Input: part model. Units: mm. Frame: model coordinates. Give positions to 0.01 mm unless a question says otherwise; leave off trailing zeros. Write each loop counter-clockwise with the first axis right and the second up, starting at its lowest first coordinate (ties: lowest second). Pieces come first, ordered by that corner, then holes. Notation, with made-up numbers: (69.5, 69.25) - (101.5, 69.25) arc R21 ccw to (101.5, 86.25) - close; hole circle Ø2 at (1, 72). An arc over 180 degrees is marked (long way). Answer as CSV lines item,"result".
```python
from build123d import *

# Parameters (mm, degrees)
F0_R     = 4.5
F0_R_2   = 3.9698540575
F1_DEPTH = 3
F0_W     = 8.4173739762
F0_H     = 21.1992750527
F0_R_3   = 3
F2_DEPTH = 3
F0_R_4   = 4.0384082605
F3_DEPTH = 3


with BuildPart() as f1:
    # F0 (on Top) → F1 (new body)
    with BuildSketch(Plane.XY):
        Polygon((0, 45.5646959671), (30.1232379104, 13.3580023242), (30.1232379104, 39.4406561247), align=None)
        with Locations((20.812695846, 33.9126698673)):
            Circle(F0_R, mode=Mode.SUBTRACT)
        Polygon((0, 45.5646959671), (30.1232379104, 39.4406561247), (30.1232379104, 60.6399311774), (0, 53.8307130337), align=None)
        with Locations((6.6491481848, 49.4420155883)):
            Circle(F0_R_2, mode=Mode.SUBTRACT)
        Polygon((0, 53.8307130337), (30.1232379104, 60.6399311774), (30.1232379104, 87.3854537311), align=None)
        with Locations((20.812695846, 66.9103562832)):
            Circle(F0_R, mode=Mode.SUBTRACT)
    extrude(amount=F1_DEPTH)

    # F0 (on Top) → F2 (join)
    with BuildSketch(Plane.XY):
        Polygon((30.1232379104, 87.3854537311), (30.1232379104, 60.6399311774), (38.5406118866, 60.6399311774), (38.5406118866, 87.3854537311), (33.5578359663, 80.3538560867), align=None)
        with Locations((34.3319248985, 50.0402936511)):
            Rectangle(F0_W, F0_H)
        with Locations((34.6380185767, 50.585233695)):
            Circle(F0_R_3, mode=Mode.SUBTRACT)
        Polygon((30.1232379104, 39.4406561247), (30.1232379104, 13.3580023242), (33.5578359663, 21.6755278666), (38.5406118866, 13.3580023242), (38.5406118866, 39.4406561247), align=None)
    extrude(amount=F2_DEPTH)

    # F0 (on Top) → F3 (join)
    with BuildSketch(Plane.XY):
        Polygon((38.5406118866, 39.4406561247), (38.5406118866, 13.3580023242), (69.6981623769, 45.5646959671), align=None)
        with Locations((46.3029742241, 33.9126698673)):
            Circle(F0_R, mode=Mode.SUBTRACT)
        Polygon((38.5406118866, 87.3854537311), (38.5406118866, 60.6399311774), (69.6981623769, 53.8307130337), align=None)
        with Locations((46.6521531343, 66.9103562832)):
            Circle(F0_R, mode=Mode.SUBTRACT)
        Polygon((38.5406118866, 60.6399311774), (38.5406118866, 39.4406561247), (69.6981623769, 45.5646959671), (69.6981623769, 53.8307130337), align=None)
        with Locations((63.4365081787, 49.4420155883)):
            Circle(F0_R_4, mode=Mode.SUBTRACT)
    extrude(amount=F3_DEPTH)


solid = f1.part
```
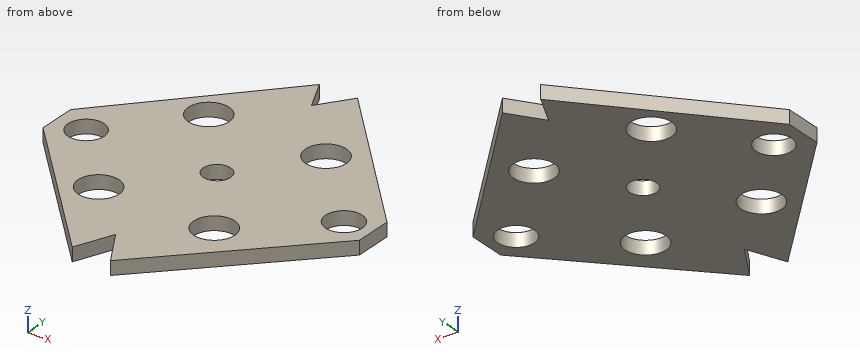
Item 1: Contact query for flat-ended pins moving along their axis: pin 1 (1 mm diameter, centred on y = 62, z = 2, fed in from +X); pin 2 (1 mm diameter, centred on y = 57.5, z = 0.5, fed in from +X). Output: stop coordinate, or through.
The answers:
pin 1,"x = 62.58"
pin 2,"x = 66.76"
Item 2: Cut plane C-C on y = 51.5. Return the cut outline in (x, z).
The answers:
outline,"(0, 0) - (3.25, 0) - (3.25, 3) - (0, 3) - close; (10.04, 0) - (31.78, 0) - (31.78, 3) - (10.04, 3) - close; (37.5, 0) - (59.96, 0) - (59.96, 3) - (37.5, 3) - close; (66.91, 0) - (69.7, 0) - (69.7, 3) - (66.91, 3) - close"
Item 3: Ray query, line 1 (Y direction, x = 48, z = 0.4); line 2 (X direction, y = 63, z = 2.4); line 3 (X direction, y = 47, z = 2.5). Return the intervals inside material, ascending. Write a range as from..to.
The answers:
line 1,"23.14..29.74, 38.08..62.62, 71.2..77.2"
line 2,"8.23..18.59, 23.04..44.43, 48.88..61.18"
line 3,"0..3.52, 9.78..60.22, 66.65..69.7"
Item 4: Cut plane A-A on y = 20. Return the cut outline in (x, z), plus the area to 3 significant figures.
The answers:
outline,"(23.91, 0) - (32.87, 0) - (32.87, 3) - (23.91, 3) - close; (34.56, 0) - (44.97, 0) - (44.97, 3) - (34.56, 3) - close"
area,"58.1 mm²"
Item 5: Cut plane B-B on z = 2.4. Return the cut outline in (x, y), plus the area to 3 significant figures.
The answers:
outline,"(0, 45.56) - (30.12, 13.36) - (33.56, 21.68) - (38.54, 13.36) - (69.7, 45.56) - (69.7, 53.83) - (38.54, 87.39) - (33.56, 80.35) - (30.12, 87.39) - (0, 53.83) - close; hole circle Ø7.94 at (6.65, 49.44); hole circle Ø9 at (20.81, 33.91); hole circle Ø9 at (20.81, 66.91); hole circle Ø6 at (34.64, 50.59); hole circle Ø9 at (46.3, 33.91); hole circle Ø9 at (46.65, 66.91); hole circle Ø8.08 at (63.44, 49.44)"
area,"2,700 mm²"
Item 6: Cut plane D-D on x = 23. Return the cut outline in (y, z).
The answers:
outline,"(20.97, 0) - (29.98, 0) - (29.98, 3) - (20.97, 3) - close; (37.85, 0) - (62.98, 0) - (62.98, 3) - (37.85, 3) - close; (70.84, 0) - (79.45, 0) - (79.45, 3) - (70.84, 3) - close"
